Work out the finished part from the listing and answer in its coordinate system (mm). A direction names the side the tool comes from. Coordinates: 2 decimals unless noted, no trailing zeros. Loops run counter-clockwise (first coordinate to the right, second up) from the corner with the lowest first, then second, coordinate; pieces in that order, holes last. Notation, with made-up numbers: (30.25, -20.75) - (84.25, -20.75) arc R12 cw to (84.25, 1.25) - close; hole circle Ø10 at (44, -14.75). An arc over 180 degrees is marked (long way). Write each question's results on one line, items separated by ' | '. Start each with the question number.
Item 1: Section B-B, the plane y = 45.5 is taken. Write down the section's boundary in (x, z).
Item 2: Consider probe 1 along X at (y, z) = (63, 6.5); probe 2 along Z at (x, y) = (18, 45.5). Determine where each line is inside the solid, lowest interval first. Write a range as [from, to].
Item 3: Section A-A, the plane z = 4 is taken. Count the separate pieces of the cut face and the enclosed holes in it, plus the area to 3 significant figures.
Item 4: A tool of negligible diameter and unlimited length cuts with its end or side. For faces 1 (the face through (12, 71.8, 4)), 2 (the face through (1.2, 19, 6)), from which of +Z, -Z, +X, -X, +Y, -Y can it reach the whole face along a straight path? Write none if from no direction.
Item 5: For a pull along X with two mould halves and no side action, classify faces 3 (the face through (12, 32.429, 5)), 4 (the face through (24.2, 35, 4)), 5 (the face through (12, 62.257, 5)), 6 (the face through (12, 36, 0)) as +X half, -X half, draft (parallel to the pull), parting line (faces both ways), or undercut.
Item 6: This flat-tipped pin is pushed along its axis until it touches: pin 1 Ø2.5 at (x, y) = (10, 36) entering from +Z. Where does it stop, or does it pass through?
from build123d import *

# Parameters (mm, degrees)
F0_W     = 24.2
F0_H     = 71.8
F1_DEPTH = 8.5
F2_W     = 21.8
F2_H     = 65.6
F3_DEPTH = 6
F5_DEPTH = 6


with BuildPart() as f1:
    # F0 (on Top) → F1 (new body)
    with BuildSketch(Plane.XY):
        with Locations((12.1, 35.9)):
            Rectangle(F0_W, F0_H)
    extrude(amount=F1_DEPTH)

    # F2 (on face) → F3 (cut)
    with BuildSketch(Plane.XY.offset(8.5)):
        with Locations((12.1, 37.8)):
            Rectangle(F2_W, F2_H)
    extrude(amount=-F3_DEPTH, mode=Mode.SUBTRACT)

    # F4 (on face) → F5 (join)
    with BuildSketch(Plane.XY.offset(2.5)):
        Polygon((11, 62.256824), (1.2, 62.256824), (1.2, 61.056824), (11, 61.056824), (12, 61.056824), (12.2, 61.056824), (13.2, 61.056824), (23, 61.056824), (23, 62.256824), (12.177438, 62.256824), (12.022562, 62.256824), align=None)
        Polygon((23, 51.514286), (23, 52.714286), (13.2, 52.714286), (12.2, 52.714286), (12, 52.714286), (11, 52.714286), (1.2, 52.714286), (1.2, 51.514286), (11, 51.514286), (12, 51.514286), (12.2, 51.514286), (13.2, 51.514286), align=None)
        Polygon((11, 43.171429), (1.2, 43.171429), (1.2, 41.971429), (11, 41.971429), (12, 41.971429), (12.2, 41.971429), (13.2, 41.971429), (23, 41.971429), (23, 43.171429), (13.2, 43.171429), (12.2, 43.171429), (12, 43.171429), align=None)
        Polygon((23, 32.428571), (23, 33.628571), (13.2, 33.628571), (12.2, 33.628571), (12, 33.628571), (11, 33.628571), (1.2, 33.628571), (1.2, 32.428571), (11, 32.428571), (12, 32.428571), (12.2, 32.428571), (13.2, 32.428571), align=None)
        Polygon((11, 24.085714), (1.2, 24.085714), (1.2, 22.885714), (11, 22.885714), (12, 22.885714), (12.2, 22.885714), (13.2, 22.885714), (23, 22.885714), (23, 24.085714), (13.2, 24.085714), (12.2, 24.085714), (12, 24.085714), align=None)
        Polygon((23, 13.342857), (23, 14.542857), (13.2, 14.542857), (12.2, 14.542857), (12, 14.542857), (11, 14.542857), (1.2, 14.542857), (1.2, 13.342857), (11, 13.342857), (12, 13.342857), (12.2, 13.342857), (13.2, 13.342857), align=None)
    extrude(amount=F5_DEPTH)


with BuildPart() as f6_1:
    # F6: copy of F1
    add(f1.part)


solid = f1.part
Answer key:
1) outline: (0, 0) - (24.2, 0) - (24.2, 8.5) - (23, 8.5) - (23, 2.5) - (1.2, 2.5) - (1.2, 8.5) - (0, 8.5) - close
2) probe 1: x = [0, 1.2], [23, 24.2] | probe 2: z = [0, 2.5]
3) separate pieces: 1 | enclosed holes: 7 | area: 464 mm^2
4) face 1: +Z, -Z, +X, -X, +Y | face 2: +Z
5) face 3: undercut | face 4: +X half | face 5: undercut | face 6: draft
6) pin 1: stops at z = 2.5
